Autodesk Inventor part; units mm, degrees
ref_plane "Work Plane1" through (40, 0, 0) normal (1, 0, 0) x (0, 1, 0)
ref_plane "XZ Plane" through (0, 0, 0) normal (0, 1, 0) x (-1, 0, 0)
ref_plane "XY Plane" through (0, 0, 0) normal (0, 0, 1) x (1, 0, 0)
sketch "Sketch1" plane through (0, 0, 0) normal (0, 1, 0) x (-1, 0, 0)
  line L0 (-35, -79) -> (35, -79)
  line L1 (55, -59) -> (55, 59)
  line L2 (35, 79) -> (-35, 79)
  line L3 (-55, 59) -> (-55, -59)
  line L4 (-55, -79) -> (55, 79) construction
  line L5 (55, -79) -> (-55, 79) construction
  arc A0 (55, 59) -> (35, 79) centre (35, 59) ccw
  arc A1 (-35, 79) -> (-55, 59) centre (-35, 59) ccw
  arc A2 (-55, -59) -> (-35, -79) centre (-35, -59) ccw
  arc A3 (35, -79) -> (55, -59) centre (35, -59) ccw
  point P0 (0, 0)
  dimension "d0" = 158
  dimension "d1" = 110
  dimension "d2" = 20
extrude "Extrusion1" add sketch "Sketch1" along normal blind 6
sketch "Sketch2" plane through (0, 0, 0) normal (0, -1, 0) x (1, 0, 0)
  line L0 (-55, -52.5) -> (55, 52.5) construction
  line L1 (55, -52.5) -> (-55, 52.5) construction
  line L2 (90.8825, 0) -> (-87.3629, 0)
  line L3 (0, 94.4084) -> (0, -106.3516)
  line L4 (-20, -52.5) -> (20, -52.5)
  line L5 (40, -32.5) -> (40, 32.5)
  line L6 (20, 52.5) -> (-20, 52.5)
  line L7 (-40, 32.5) -> (-40, -32.5)
  line L8 (-40, -52.5) -> (40, 52.5) construction
  line L9 (40, -52.5) -> (-40, 52.5) construction
  line L10 (40, 52.5) -> (41.9971, 52.5)
  line L11 (40, -52.5) -> (41.9971, -52.5)
  line L12 (40, 52.5) -> (40, 71.6594)
  line L13 (40, -52.5) -> (40, -69.6689)
  arc A0 (40, 32.5) -> (20, 52.5) centre (20, 32.5) ccw
  arc A1 (-20, 52.5) -> (-40, 32.5) centre (-20, 32.5) ccw
  arc A2 (-40, -32.5) -> (-20, -52.5) centre (-20, -32.5) ccw
  arc A3 (20, -52.5) -> (40, -32.5) centre (20, -32.5) ccw
  point P0 (0, 0)
  dimension "d23" = 52.5
  dimension "d25" = 40
  dimension "d26" = 20
extrude "Extrusion2" add sketch "Sketch2" along normal blind 18
sketch "Sketch3" plane through (0, 6, 0) normal (0, 1, 0) x (1, 0, 0)
  circle A0 centre (-37.5, -55) radius 5
  circle A1 centre (37.5, -55) radius 5
  line L0 (-35.6722, 52.5) -> (-19.5402, 52.5)
  line L1 (0, 83.5001) -> (0, -85.7722)
  line L2 (-75.2069, 0) -> (80.66, 0)
  line L3 (-37.5, -55) -> (37.5, -55)
  line L4 (-37.5, -55) -> (-37.5, -56.2391)
  line L5 (37.5, -55) -> (37.5, -56.2391)
  circle A2 centre (-37.5, 55) radius 5
  circle A3 centre (37.5, 55) radius 5
  point P0 (0, 0)
  dimension "d15" = 37.5
  dimension "d16" = 37.5
  dimension "d17" = 55
  dimension "d20" = 10
  dimension "d21" = 10
extrude "Extrusion3" cut sketch "Sketch3" against normal blind 6
ref_plane "Work Plane1" through (40, 0, 0) normal (1, 0, 0) x (0, 1, 0)
sketch "Sketch4" plane through (40, 0, 0) normal (1, 0, 0) x (0, 1, 0)
  arc A0 (-112.3326, 65.8559) -> (-126.6551, 28.523) centre (-119, 47) ccw
  circle A1 centre (-119, 47) radius 62.5
  line L0 (-18, -32.5) -> (-18, 32.5)
  line L1 (6, 59) -> (6, -59)
  line L2 (63.9503, 0) -> (-247.3631, 0)
  line L3 (-119, 47) -> (-214.4005, 47)
  line L4 (-18, -32.5) -> (-62.0453, -32.5)
  line L5 (-18, 32.5) -> (-18, -32.5)
  line L6 (-18, 32.5) -> (-112.3326, 65.8559)
  line L7 (-62.0453, -32.5) -> (-126.6551, 28.523)
  point P0 (0, 0)
  point P1 (-131.6551, 40.5657)
  dimension "d28" = 40
  dimension "d29" = 125
  dimension "d30" = 125
  dimension "d31" = 47
extrude "Extrusion4" add sketch "Sketch4" against normal blind 17.5 contours L6 A1 L2 L7 A0 | L6 L0 L2 A1 | L2 L0 L4 L7 A1 | A1 L7 L2 picked at (-85.1463, -0.9198)
mirror "Mirror1" about plane through (0, 0, 0) normal (1, 0, 0) of "Extrusion4"
sketch "Sketch5" plane through (40, 0, 32.5) normal (1, 0, 0) x (0, 0, -1)
  arc A0 (-33.3559, -112.3326) -> (3.977, -126.6551) centre (-14.5, -119) ccw
  circle A1 centre (-14.5, -119) radius 7.5
  point P0 (32.5, 0)
  dimension "d35" = 15
extrude "Extrusion5" cut sketch "Sketch5" against normal through all
properties part number "Plate2" material "Polyethylene, High Density"
Part model, mm, in its own coordinate system. A direction names the side the tool comes from. Give positions to 0.01 mm unless a question says otherwise; leave off trailing zeros. Loops run counter-clockwise (first coordinate to the right, second up) from the corner with the lowest first, then second, coordinate; pieces in that order, holes last. Notation, with made-up numbers: (62, -25) -> (95, -25) arc R17 ccw to (95, 3) -> close; hole circle Ø6 at (6.5, 71). An arc over 180 degrees is marked (long way). Write each question's results on one line, items separated by ' | '. Start each with the question number.
Q1. Pin check, flat tips, straight feed: P1, Ø10, axis at x = -38.5, y = -86, coming from the +Z side; P2, Ø14, axis at x = -29, y = -43.5, coming from the -Z side; P3, Ø12, axis at x = 31, z = -23.5, coming from the -Y side. Stop position of each tip, or through.
Q2. Which spindle directions (+Z, -Z, +X, -X, +Y, -Y) get a long thin tool onto all of the face, cutting with end or side? Do faces 1 (the face through (0, -9, 52.5)), 2 (the face through (34.297, -8.874, -46.486)), 3 (the face through (0, -9, -52.5)), 4 (the face through (22.5, -66, 18)). Say none if no direction does.
Q3. Band-saw the part on B-B on x = 37.5. List the corners of the cut face in (y, z).
Q4. Band-saw the part on C-C on y = -37. List the corners of the cut face in (x, z), plus the area to 3 significant figures.
Q5. Band-saw the part on A-A on z = -55. List the corners of the cut face in (x, y), plus the area to 3 significant figures.
Q6. Wall check: L1, parallel to X at y = 3.4, z = 55; L2, parallel to X at y = -81.5, z = 34; L3, parallel to Z at x = -37, y = 2. Give the ranges that are in metal, low to high.
Q7. Pull direction Y, two halves, no side cores. Call faces 5 (the face through (1, 6, 1)), 6 (the face through (31, -40, -32.5)), 7 (the face through (-31.127, -125.654, 43.539)), 8 (the face through (-31.373, -94.802, -1.561)): +Y half, -Y half, draft (parallel to the pull), parting line (faces both ways), or undercut.
Q8. Band-saw the part on D-D on y = -119. List the corners of the cut face in (x, z).
Results are:
1) P1: stops at z = 58.31 | P2: stops at z = -32.5 | P3: stops at y = -77.93
2) face 1: +Z, +X, -X, -Y | face 2: -Z, +X, -Y | face 3: -Z, +X, -X, -Y | face 4: +Z, -Z, -Y
3) outline: (-126.66, 28.52) -> (-62.05, -32.5) -> (-18, -32.5) -> (-18, -42.18) -> (0, -42.18) -> (0, -50) -> (6, -50) -> (6, 50) -> (0, 50) -> (0, 42.18) -> (-18, 42.18) -> (-18, 32.5) -> (-112.33, 65.86) arc R20 ccw to start; (0, -78.84) -> (6, -78.84) -> (6, -60) -> (0, -60) -> close; (0, 60) -> (6, 60) -> (6, 78.84) -> (0, 78.84) -> close; hole circle Ø15 at (-119, 47)
4) outline: (-40, -32.5) -> (-22.5, -32.5) -> (-22.5, 39.22) -> (-40, 39.22) -> close; (22.5, -32.5) -> (40, -32.5) -> (40, 39.22) -> (22.5, 39.22) -> close | area: 2,510 mm²
5) outline: (-55, 0) -> (-42.5, 0) -> (-42.5, 6) -> (-55, 6) -> close; (-32.5, 0) -> (32.5, 0) -> (32.5, 6) -> (-32.5, 6) -> close; (42.5, 0) -> (55, 0) -> (55, 6) -> (42.5, 6) -> close | area: 540 mm²
6) L1: x = -55 to -42.5, -32.5 to 32.5, 42.5 to 55 | L2: x = -40 to -22.5, 22.5 to 40 | L3: z = -78.9 to -59.97, -50.03 to 50.03, 59.97 to 78.9
7) face 5: +Y half | face 6: draft | face 7: undercut | face 8: -Y half
8) outline: (-40, 21.29) -> (-22.5, 21.29) -> (-22.5, 39.5) -> (-40, 39.5) -> close; (-40, 54.5) -> (-22.5, 54.5) -> (-22.5, 67) -> (-40, 67) -> close; (22.5, 21.29) -> (40, 21.29) -> (40, 39.5) -> (22.5, 39.5) -> close; (22.5, 54.5) -> (40, 54.5) -> (40, 67) -> (22.5, 67) -> close
